Geometry: final body of the model. Coordinates: model frame, mm. Coordinates: 2 decimals unless noted, no trailing zeros. Write each loop counter-clockwise with the first axis right and the second up, starting at its lowest first coordinate (ties: lowest second). Pieces come first, ordered by that corner, then holes. Notation, with made-up numbers: (12.5, 35) - (33.5, 35) arc R13 ccw to (33.5, 46) - close; hole circle Ø2 at (65, -38). An arc over 180 degrees is marked (long way). Answer as a JSON object with one key per item and string values. Group by question number.
Item 1: Section A-A on x = -36. Return loops of the section in (y, z).
Item 2: Line query: line 1 along Z through (x, y) = (-41, 2.3); line 2 along X through (y, z) = (0.2, 28); line 3 along Z through (x, y) = (23.5, 1.85). Output: solid intervals per line, ascending. Write a range as from..to.
Item 3: First-contact query: pin 1 Ø1.5 at (x, z) = (93, 29.5) entering from -Y; pin 2 Ø1.5 at (x, y) = (-1.5, 1.5) entering from +Z; pin 3 Ø0.9 at (x, y) = (-181, 1.5) entering from -Z; pin 4 Ø1.5 at (y, z) = (2, 149.5) entering from -X. Flat tips, straight axial feed; report the tip coordinate or a pass-through.
Item 4: Section C-C on y = 1.8. State how many separate pieces and enclosed holes the cut face has, and give its area (3 significant figures).
Item 5: Section B-B on z = -86.5. Return loops of the section in (x, y).
Item 6: Section D-D on x = -174. Return loops of the section in (y, z).
```python
from build123d import *

# Parameters (mm, degrees)
SKETCH1_R           = 1
SKETCH1_R_2         = 10
BOSS_EXTRUDE1_DEPTH = 3


with BuildPart() as part:
    # Sketch1 → Boss-Extrude1 (new body)
    with BuildSketch(Plane(origin=(0, 0, 0), x_dir=(1, 0, 0), z_dir=(0, 1, 0))):
        Polygon((-111.790938792, 69.703810947), (-111.790938792, 82.203810947), (-60.290938792, 82.203810947), (-60.290938792, 112.203810947), (-20.290938792, 112.203810947), (-20.290938792, 82.203810947), (31.209061208, 82.203810947), (31.209061208, 69.703810947), (134.709061208, 69.703810947), (134.709061208, -115.296189053), (31.209061208, -115.296189053), (31.209061208, -127.796189053), (-20.290938792, -127.796189053), (-20.290938792, -157.796189053), (-60.290938792, -157.796189053), (-60.290938792, -127.796189053), (-111.790938792, -127.796189053), (-111.790938792, -115.296189053), (-215.290938792, -115.296189053), (-215.290938792, 69.703810947), align=None)
        with Locations((-5.290938792, -47.796189053)):
            Circle(SKETCH1_R, mode=Mode.SUBTRACT)
        with Locations((-5.290938792, 2.203810947)):
            Circle(SKETCH1_R, mode=Mode.SUBTRACT)
        with Locations((-62.290938792, -53.796189053)):
            Circle(SKETCH1_R, mode=Mode.SUBTRACT)
        with Locations((-62.290938792, 8.203810947)):
            Circle(SKETCH1_R, mode=Mode.SUBTRACT)
        with Locations((-40.290938792, 92.203810947)):
            Circle(SKETCH1_R_2, mode=Mode.SUBTRACT)
        with Locations((-40.290938792, -137.796189053)):
            Circle(SKETCH1_R_2, mode=Mode.SUBTRACT)
        with Locations((114.709061208, -22.796189053)):
            Circle(SKETCH1_R_2, mode=Mode.SUBTRACT)
        with Locations((-195.290938792, -22.796189053)):
            Circle(SKETCH1_R_2, mode=Mode.SUBTRACT)
    extrude(amount=BOSS_EXTRUDE1_DEPTH)


solid = part.part
```
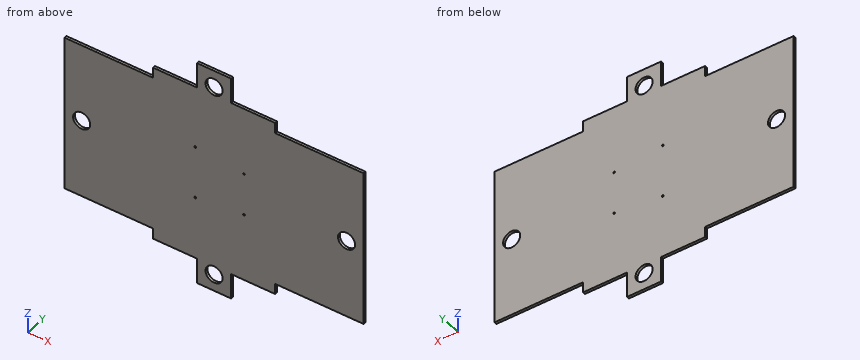
Checks:
{
 "1": {"outline": "(0, -112.2) - (3, -112.2) - (3, -101.24) - (0, -101.24) - close; (0, -83.17) - (3, -83.17) - (3, 128.76) - (0, 128.76) - close; (0, 146.83) - (3, 146.83) - (3, 157.8) - (0, 157.8) - close"},
 "2": {"line 1": "-112.2..-102.18, -82.23..127.82, 147.77..157.8", "line 2": "-215.29..-203.83, -186.75..106.17, 123.25..134.71", "line 3": "-82.2..127.8"},
 "3": {"pin 1": "y = 0", "pin 2": "z = 127.8", "pin 3": "z = -69.7", "pin 4": "x = -60.29"},
 "4": {"separate pieces": "1", "enclosed holes": "8", "area": "69,500 mm^2"},
 "5": {"outline": "(-60.29, 0) - (-48.5, 0) - (-48.5, 3) - (-60.29, 3) - close; (-32.08, 0) - (-20.29, 0) - (-20.29, 3) - (-32.08, 3) - close"},
 "6": {"outline": "(0, -69.7) - (3, -69.7) - (3, 115.3) - (0, 115.3) - close"}
}
